Read the model definition and answer for the solid it produces. Units are mm, in the model's axes. A direction names the side the tool comes from. Give positions to 0.01 mm unless a question says otherwise; leave off trailing zeros. Order: outer loops, then holes, each group sorted by start corner. A loop starts at its lowest first (then second) coordinate and runs counter-clockwise, first axis right, second up. Notation, with made-up numbers: (68, 23.25) - (119, 23.25) arc R8 cw to (119, 36.25) - close; hole circle Ø7 at (-30, -25). An arc over 180 degrees is marked (long way). Use a Markdown table: item, result. Add a question column.
1. Consider L1, parallel to X at y = -2.5, z = -27.5; L2, parallel to Z at x = 31, y = 11; L3, parallel to X at y = -32.5, z = 23. Determine where each line is inside the solid, lowest interval first.
2. A cutting plane is placed at B-B on y = -21. Determine the outline of the cut face in (x, z), and give its area (3 significant figures).
3. A cutting plane is placed at C-C on x = 39.5. Determine the outline of the cut face in (y, z).
4. A cutting plane is placed at A-A on x = 12. Determine the outline of the cut face in (y, z).
5. Which of the six approach directions +Z, -Z, +X, -X, +Y, -Y give full straight-line access (tool end or side, diameter ignored) to faces 4 (the flat face through (3.742, 0, -25)), 5 (the flat face through (30, -6, 48.63)), 6 (the flat face through (13.742, 0, -25)), 7 (the flat face through (9, -3.312, -25)), 8 (the flat face through (56, 2.688, -25))?
6. Flat-ended cylindrical pins translate along their axes: P1, Ø12, axis at y = 9, z = 39, coming from the +X side; P2, Ø3, axis at x = 7.5, z = -22.5, coming from the -Y side; P3, Ø1.5, axis at x = 38.5, y = 13, coming from the -Z side. Find the tip coordinate at first contact, or state that the pin passes through.
7. For a pull along X with two mould halves and no side action, classify faces 1 (the flat face through (0, -6, 16)), 2 (the flat face through (30, -37.396, 15)), 3 (the flat face through (51.006, 0, -25)) as released by +X, released by -X, zero draft, split by the parting line, or undercut.
```python
from build123d import *

# Parameters (mm, degrees)
F0_W     = 63.5
F0_H     = 66.04
F1_DEPTH = 60.96
F2_R     = 5.08
F3_W     = 10
F3_H     = 6
F4_DEPTH = 15


with BuildPart() as f1:
    # F0 (on Right) → F1 (new body)
    with BuildSketch(Plane.YZ):
        with Locations((-5.645866, 15.610142)):
            Rectangle(F0_W, F0_H)
    extrude(amount=F1_DEPTH)

    # F2
    f2_edges = [f1.edges().sort_by_distance(p)[0] for p in [
        (60.96, -37.395866, 15.610142),
        (60.96, 26.104134, 15.610142),
        (0, -37.395866, 15.610142),
        (0, 26.104134, 15.610142),
    ]]
    fillet(f2_edges, radius=F2_R)

    # F3 (on face) → F4 (join)
    with BuildSketch(Plane(origin=(0, 0, -17.409858), x_dir=(1, 0, 0), z_dir=(0, 0, -1))):
        with Locations((8.742291, 0.311744)):
            Rectangle(F3_W, F3_H)
        with Locations((56.006265, 0.311744)):
            Rectangle(F3_W, F3_H)
    extrude(amount=F4_DEPTH)


solid = f1.part
```
Output values:
| question | item | result |
|---|---|---|
| 1 | L1 | 3.74 to 13.74, 51.01 to 61.01 |
| 1 | L2 | -17.41 to 48.63 |
| 1 | L3 | 0 to 60.96 |
| 2 | outline | (0, -17.41) - (60.96, -17.41) - (60.96, 48.63) - (0, 48.63) - close |
| 2 | area | 4,030 mm² |
| 3 | outline | (-37.4, -17.41) - (26.1, -17.41) - (26.1, 48.63) - (-37.4, 48.63) - close |
| 4 | outline | (-37.4, -17.41) - (-3.31, -17.41) - (-3.31, -32.41) - (2.69, -32.41) - (2.69, -17.41) - (26.1, -17.41) - (26.1, 48.63) - (-37.4, 48.63) - close |
| 5 | face 4 | -Z, -X, +Y, -Y |
| 5 | face 5 | +Z, +X, -X, +Y, -Y |
| 5 | face 6 | -Z, +Y, -Y |
| 5 | face 7 | -Z, +X, -X, -Y |
| 5 | face 8 | -Z, +X, -X, +Y |
| 6 | P1 | x = 60.96 |
| 6 | P2 | y = -3.31 |
| 6 | P3 | z = -17.41 |
| 7 | face 1 | released by -X |
| 7 | face 2 | zero draft |
| 7 | face 3 | undercut |
